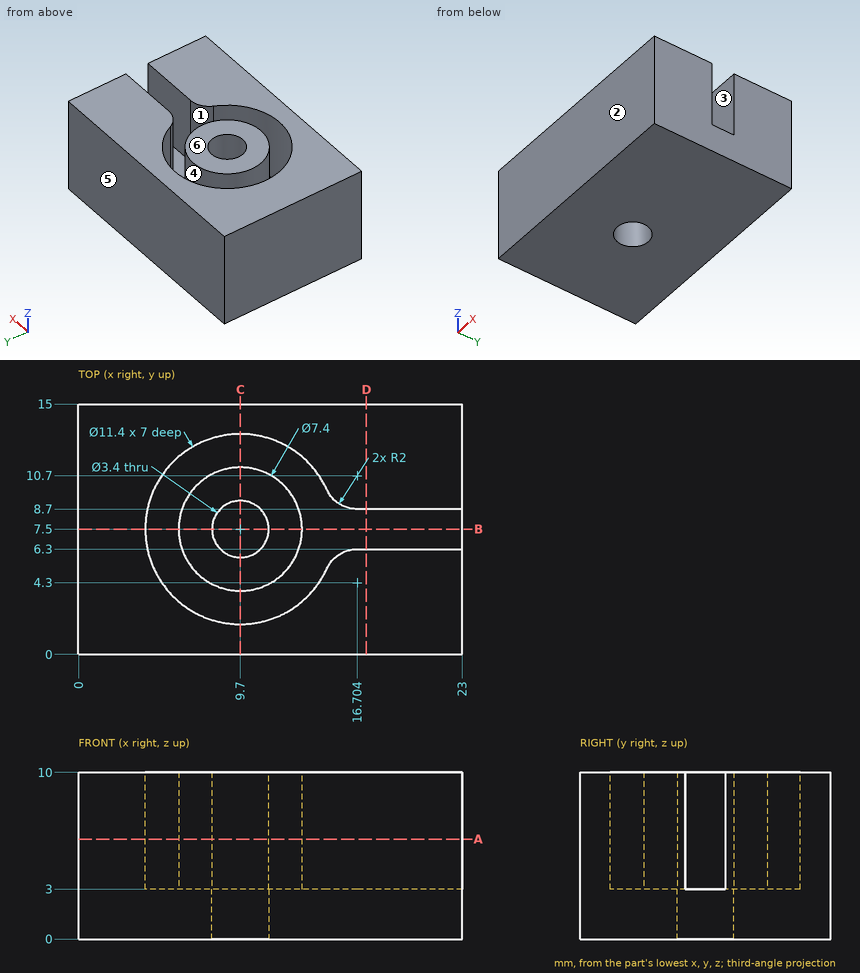
Verification items for this drawing (mm, ordinates from the low corner). A direction names the side the tool comes from. Coordinates: 2 decimals unless noted, no trailing zeros. Order: outer loops, then holes, each group sorted by start corner. A loop starts at its lowest first (then second) coordinate and runs counter-clockwise, first axis right, second up. Notation, with made-up numbers: (57.25, 57) -> (80.25, 57) arc R35 cw to (80.25, 90) -> close; hole circle Ø9 at (-31.5, 32). An arc over 180 degrees is marked (long way). Answer as CSV lines item,"result". Start each with the question number.
1) Cross-section at D-D, the plane x = 17.25. Record the boundary of the cut face in (y, z).
2) Cross-section at B-B, the plane y = 7.5. Record the boundary of the cut face in (x, z), then the cut area to 3 significant figures.
3) Set-up check for the marked faces 1, 2 and 3: record each of +Z, -Z, +X, -X, +Y, -Y from which the full face is reachable in a straight line by a thin tool's end or side.
4) Gauge pin test, flat end, axial feed: pin 1 Ø4.5 at (x, y) = (9.7, 7.5) entering from -Z. Record the tip position at first contact, or that the pin passes through.
5) Material ranges on L1, parallel to Y at x = 9.7, z = 5.25; L2, parallel to Y at x = 21.75, z = 7.5; L3, parallel to Y at x = 6.75, z = 8.75 (1 decimal), recorded low to high. Write a range as [from, to].
6) Release check for a two-part mould opening along Y. For the marked faces 4, 5 and 6 record: released by +Y, released by -Y, zero draft, split by the parting line, or undercut.
7) Cross-section at A-A, the plane z = 6. Record the boundary of the cut face in (x, y) (1 decimal).
8) Cross-section at C-C, the plane x = 9.7. Record the boundary of the cut face in (y, z).
Conclusion:
1,outline,"(0, 0) -> (15, 0) -> (15, 10) -> (8.7, 10) -> (8.7, 3) -> (6.3, 3) -> (6.3, 10) -> (0, 10) -> close"
2,outline,"(0, 0) -> (8, 0) -> (8, 10) -> (6, 10) -> (6, 3) -> (4, 3) -> (4, 10) -> (0, 10) -> close; (11.4, 0) -> (23, 0) -> (23, 3) -> (13.4, 3) -> (13.4, 10) -> (11.4, 10) -> close"
2,area,"115 mm²"
3,face 1,"+Z"
3,face 2,"+Z, -Z, +X, -X, -Y"
3,face 3,"+Z, +X"
4,pin 1,"stops at z = 0"
5,L1,"y = [0, 1.8], [3.8, 5.8], [9.2, 11.2], [13.2, 15]"
5,L2,"y = [0, 6.3], [8.7, 15]"
5,L3,"y = [0, 2.6], [5.3, 9.7], [12.4, 15]"
6,face 4,"undercut"
6,face 5,"released by +Y"
6,face 6,"zero draft"
7,outline,"(0, 0) -> (23, 0) -> (23, 6.3) -> (16.7, 6.3) arc R2 ccw to (14.9, 5.1) arc R5.7 cw (long way) to (14.9, 9.9) arc R2 ccw to (16.7, 8.7) -> (23, 8.7) -> (23, 15) -> (0, 15) -> close; circle Ø7.4 at (9.7, 7.5); hole circle Ø3.4 at (9.7, 7.5)"
8,outline,"(0, 0) -> (5.8, 0) -> (5.8, 10) -> (3.8, 10) -> (3.8, 3) -> (1.8, 3) -> (1.8, 10) -> (0, 10) -> close; (9.2, 0) -> (15, 0) -> (15, 10) -> (13.2, 10) -> (13.2, 3) -> (11.2, 3) -> (11.2, 10) -> (9.2, 10) -> close"
